```python
from build123d import *

# Parameters (mm, degrees)
F0_R     = 2.219223
F0_R_2   = 1.529807
F0_R_3   = 2.219078
F0_R_4   = 2.227919
F0_R_5   = 1.528278
F0_R_6   = 2.219557
F1_DEPTH = 6.35
F2_R     = 1.529807
F2_R_2   = 1.530286
F2_R_3   = 1.528278
F3_DEPTH = 3.175


with BuildPart() as f1:
    # F0 (on Front) → F1 (new body)
    with BuildSketch(Plane.XZ):
        with BuildLine():
            Line((54.2656, 41.2496), (-53.6194, 41.2496))
            ThreePointArc((-53.6194, 41.2496), (-55.864464, 40.319664), (-56.7944, 38.0746))
            Line((-56.7944, 38.0746), (-56.7944, -32.3604))
            ThreePointArc((-56.7944, -32.3604), (-56.236438, -33.707438), (-54.8894, -34.2654))
            Line((-54.8894, -34.2654), (-53.6194, -34.2654))
            ThreePointArc((-53.6194, -34.2654), (-52.272362, -34.823362), (-51.7144, -36.1704))
            Line((-51.7144, -36.1704), (-51.7144, -38.7104))
            ThreePointArc((-51.7144, -38.7104), (-50.970451, -40.506451), (-49.1744, -41.2504))
            Line((-49.1744, -41.2504), (54.2656, -41.2504))
            ThreePointArc((54.2656, -41.2504), (56.061651, -40.506451), (56.8056, -38.7104))
            Line((56.8056, -38.7104), (56.8056, -35.401342))
            ThreePointArc((56.8056, -35.401342), (56.40343, -33.854721), (55.298806, -32.699913))
            Line((55.298806, -32.699913), (52.812394, -31.164487))
            ThreePointArc((52.812394, -31.164487), (51.70777, -30.009679), (51.3056, -28.463058))
            Line((51.3056, -28.463058), (51.3056, 28.811881))
            ThreePointArc((51.3056, 28.811881), (51.761511, 30.451144), (52.998313, 31.619629))
            Line((52.998313, 31.619629), (55.112887, 32.735971))
            ThreePointArc((55.112887, 32.735971), (56.349689, 33.904456), (56.8056, 35.543719))
            Line((56.8056, 35.543719), (56.8056, 38.7096))
            ThreePointArc((56.8056, 38.7096), (56.061651, 40.505651), (54.2656, 41.2496))
        make_face()
        with Locations((-52.7944, -29.7504)):
            Circle(F0_R, mode=Mode.SUBTRACT)
        with Locations((-44.0944, -20.3454)):
            Circle(F0_R_2, mode=Mode.SUBTRACT)
        with Locations((53.3056, -36.9504)):
            Circle(F0_R_3, mode=Mode.SUBTRACT)
        with Locations((-52.7944, 33.2496)):
            Circle(F0_R_4, mode=Mode.SUBTRACT)
        with Locations((-44.0944, 33.2486)):
            Circle(F0_R_5, mode=Mode.SUBTRACT)
        with BuildLine():
            ThreePointArc((43.330965, -20.8534), (41.843067, -24.445502), (38.250965, -25.9334))
            Line((38.250965, -25.9334), (-33.205545, -25.9334))
            ThreePointArc((-33.205545, -25.9334), (-35.543803, -25.363272), (-37.357216, -23.780861))
            Line((-37.357216, -23.780861), (-41.896071, -17.343939))
            ThreePointArc((-41.896071, -17.343939), (-42.586759, -15.952042), (-42.8244, -14.416478))
            Line((-42.8244, -14.416478), (-42.8244, 14.03877))
            ThreePointArc((-42.8244, 14.03877), (-42.693554, 15.184314), (-42.307758, 16.270847))
            Line((-42.307758, 16.270847), (-32.787406, 35.734677))
            ThreePointArc((-32.787406, 35.734677), (-30.913607, 37.812203), (-28.224048, 38.5826))
            Line((-28.224048, 38.5826), (38.250965, 38.5826))
            ThreePointArc((38.250965, 38.5826), (41.843067, 37.094702), (43.330965, 33.5026))
            Line((43.330965, 33.5026), (43.330965, 27.081825))
            ThreePointArc((43.330965, 27.081825), (43.19507, 25.91468), (42.794655, 24.80998))
            Line((42.794655, 24.80998), (40.692275, 20.60522))
            ThreePointArc((40.692275, 20.60522), (40.29186, 19.50052), (40.155965, 18.333375))
            Line((40.155965, 18.333375), (40.155965, -5.684175))
            ThreePointArc((40.155965, -5.684175), (40.29186, -6.85132), (40.692275, -7.95602))
            Line((40.692275, -7.95602), (42.794655, -12.16078))
            ThreePointArc((42.794655, -12.16078), (43.19507, -13.26548), (43.330965, -14.432625))
            Line((43.330965, -14.432625), (43.330965, -20.8534))
        make_face(mode=Mode.SUBTRACT)
        with BuildLine():
            ThreePointArc((43.330965, 7.981886), (44.413041, 7.533676), (44.861251, 6.4516))
            ThreePointArc((44.861251, 6.4516), (44.413041, 5.369524), (43.330965, 4.921314))
            ThreePointArc((43.330965, 4.921314), (41.800678, 6.4516), (43.330965, 7.981886))
        make_face(mode=Mode.SUBTRACT)
        with Locations((53.3056, 36.7496)):
            Circle(F0_R_6, mode=Mode.SUBTRACT)
    extrude(amount=-F1_DEPTH)

    # F2 (on face) → F3 (cut)
    with BuildSketch(Plane(origin=(0, 6.35, 0), x_dir=(-1, 0, 0), z_dir=(0, 1, 0))):
        with BuildLine():
            Line((-47.775965, -29.4894), (48.1584, -29.4894))
            ThreePointArc((48.1584, -29.4894), (49.505438, -28.931438), (50.0634, -27.5844))
            Line((50.0634, -27.5844), (50.0634, 41.2496))
            Line((50.0634, 41.2496), (-49.680965, 41.2496))
            Line((-49.680965, 41.2496), (-49.680965, -27.5844))
            ThreePointArc((-49.680965, -27.5844), (-49.123003, -28.931438), (-47.775965, -29.4894))
        make_face()
        with Locations((44.0944, -20.3454)):
            Circle(F2_R, mode=Mode.SUBTRACT)
        with Locations((-43.330965, 6.4516)):
            Circle(F2_R_2, mode=Mode.SUBTRACT)
        with BuildLine():
            ThreePointArc((-40.692275, -7.95602), (-40.29186, -6.85132), (-40.155965, -5.684175))
            Line((-40.155965, -5.684175), (-40.155965, 18.333375))
            ThreePointArc((-40.155965, 18.333375), (-40.29186, 19.50052), (-40.692275, 20.60522))
            Line((-40.692275, 20.60522), (-42.794655, 24.80998))
            ThreePointArc((-42.794655, 24.80998), (-43.19507, 25.91468), (-43.330965, 27.081825))
            Line((-43.330965, 27.081825), (-43.330965, 33.5026))
            ThreePointArc((-43.330965, 33.5026), (-41.843067, 37.094702), (-38.250965, 38.5826))
            Line((-38.250965, 38.5826), (28.224048, 38.5826))
            ThreePointArc((28.224048, 38.5826), (30.913607, 37.812203), (32.787406, 35.734677))
            Line((32.787406, 35.734677), (42.307758, 16.270847))
            ThreePointArc((42.307758, 16.270847), (42.693554, 15.184314), (42.8244, 14.03877))
            Line((42.8244, 14.03877), (42.8244, -14.416478))
            ThreePointArc((42.8244, -14.416478), (42.586759, -15.952042), (41.896071, -17.343939))
            Line((41.896071, -17.343939), (37.357216, -23.780861))
            ThreePointArc((37.357216, -23.780861), (35.543803, -25.363272), (33.205545, -25.9334))
            Line((33.205545, -25.9334), (-38.250965, -25.9334))
            ThreePointArc((-38.250965, -25.9334), (-41.843067, -24.445502), (-43.330965, -20.8534))
            Line((-43.330965, -20.8534), (-43.330965, -14.432625))
            ThreePointArc((-43.330965, -14.432625), (-43.19507, -13.26548), (-42.794655, -12.16078))
            Line((-42.794655, -12.16078), (-40.692275, -7.95602))
        make_face(mode=Mode.SUBTRACT)
        with Locations((44.0944, 33.2486)):
            Circle(F2_R_3, mode=Mode.SUBTRACT)
    extrude(amount=-F3_DEPTH, mode=Mode.SUBTRACT)


solid = f1.part
```
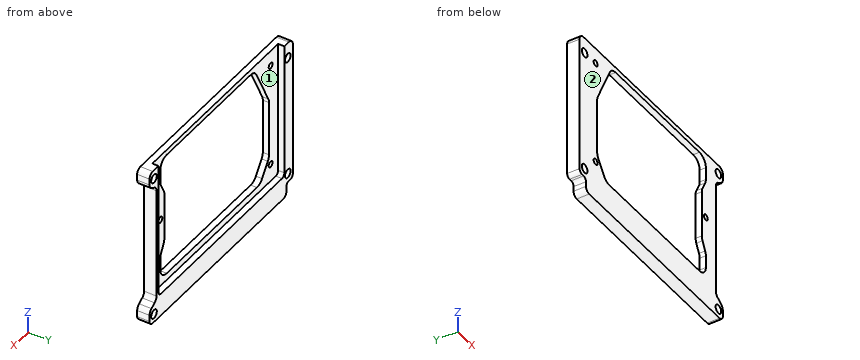
Geometry check sheet. Reference: the model listing, model coordinates, mm. Face numbers are marked on the shaded views. Give positions to 0.01 mm unless a question says otherwise; leave off trailing zeros. Write each loop counter-clockwise with the first axis right and the second up, starting at its lowest first coordinate (ties: lowest second). Pieces come first, ordered by that corner, then holes.
1) Section check B-B, the plane x = -9. Record the boundary of the cut face in (y, z) (3 decimals).
2) Material ranges on L1, parallel to Z at x = -44, y = 1; L2, parallel to X at y = 3.25, z = -1.5; L3, parallel to Z at x = -15, y = 0.75, recorded low to high.
3) Section check A-A, the plane z = -1.5. Record the boundary of the cut face in (x, y) (3 decimals), and give its area (3 significant figures).
4) Gauge pin test, flat ends, axial feed: pin 1 (2 mm diameter, centred on x = 18, y = 4, fed in from +Z); pin 2 (1.5 mm diameter, centred on x = 27, z = -24.5, fed in from +Y); pin 3 (1.3 mm diameter, centred on y = 2, z = -38, fed in from -X); pin 4 (2 mm diameter, centred on x = -44.5, z = -23, fed in from +Y) (3 decimals). Record the tip position at first contact, or that the pin passes through.
5) Section check C-C, the plane y = 4.25. State how many separate pieces and enclosed holes the cut face has, and give its area (3 significant figures).
6) Release check for a two-part mould opening along X. For the marked faces 1 and 2 record: pulls with the +X half, pulls with the -X half, needs draft (parallel to the pull), parting line crosses it, or undercut.
Computed:
1. outline: (0, -41.25) - (6.35, -41.25) - (6.35, -29.489) - (3.175, -29.489) - (3.175, -25.933) - (0, -25.933) - close; (0, 38.583) - (3.175, 38.583) - (3.175, 41.25) - (0, 41.25) - close
2. L1: z = -41.25 to -21.87, -18.82 to 31.72, 34.77 to 41.25
2. L2: x = -56.79 to -50.06, 49.68 to 51.31
2. L3: z = -41.25 to -25.93, 38.58 to 41.25
3. outline: (-56.794, 0) - (-42.824, 0) - (-42.824, 3.175) - (-50.063, 3.175) - (-50.063, 6.35) - (-56.794, 6.35) - close; (40.156, 0) - (51.306, 0) - (51.306, 6.35) - (49.681, 6.35) - (49.681, 3.175) - (40.156, 3.175) - close
3. area: 106 mm2
4. pin 1: stops at z = 41.25
4. pin 2: passes through
4. pin 3: stops at x = -51.71
4. pin 4: stops at y = 3.175
5. separate pieces: 1
5. enclosed holes: 4
5. area: 1,860 mm2
6. face 1: undercut
6. face 2: needs draft
